Input: part model. Units: mm. Frame: model coordinates. A direction names the side the tool comes from. Coordinates: 2 decimals unless noted, no trailing zeros. Loops run counter-clockwise (first coordinate to the right, second up) from the corner with the lowest first, then second, coordinate; pieces in that order, holes last. Notation, with made-up numbers: (-4, -7) - (34, -7) arc R21 ccw to (34, 26) - close; hole circle Ø5 at (-14, 87.5). An arc over 180 degrees is marked (long way). Use one line per item in the form item = value.
from build123d import *

# Parameters (mm, degrees)
SKETCH1_W           = 0.508
SKETCH1_H           = 46.99
BOSS_EXTRUDE1_DEPTH = 6.35
SKETCH2_R           = 1
CUT_EXTRUDE1_DEPTH  = 6.35
SKETCH3_R           = 1
CUT_EXTRUDE2_DEPTH  = 6.35
SKETCH4_R           = 1
CUT_EXTRUDE3_DEPTH  = 2.54


with BuildPart() as part:
    # Sketch1 → Boss-Extrude1 (new body)
    with BuildSketch(Plane.XY):
        with Locations((0.254, 23.495)):
            Rectangle(SKETCH1_W, SKETCH1_H)
        Polygon((0, 46.99), (0.508, 46.99), (5.588, 67.31), (5.08, 67.31), align=None)
        Polygon((5.588, -20.32), (0.508, 0), (0, 0), (5.08, -20.32), align=None)
    extrude(amount=BOSS_EXTRUDE1_DEPTH)

    # Sketch2 → Cut-Extrude1 (cut)
    with BuildSketch(Plane.ZY):
        with Locations((3.175, 3.048)):
            Circle(SKETCH2_R)
        with Locations((3.175, 15.748)):
            Circle(SKETCH2_R)
        with Locations((3.175, 43.942)):
            Circle(SKETCH2_R)
        with Locations((3.175, 31.242)):
            Circle(SKETCH2_R)
    extrude(amount=-CUT_EXTRUDE1_DEPTH, mode=Mode.SUBTRACT)

    # Sketch3 → Cut-Extrude2 (cut)
    with BuildSketch(Plane(origin=(-11.056470588, 2.764117647, 0), x_dir=(0, 0, 1), z_dir=(-0.9701425001453319, 0.24253562503633325, 0))):
        with Locations(Location((3.175, 63.53237266, 0), (0, 0, 270))):
            Circle(SKETCH3_R)
    extrude(amount=-CUT_EXTRUDE2_DEPTH, mode=Mode.SUBTRACT)

    # Sketch4 → Cut-Extrude3 (cut)
    with BuildSketch(Plane(origin=(0.478117647, 0.119529412, 0), x_dir=(0, 0, -1), z_dir=(0.9701425001453319, 0.24253562503633308, 0))):
        with Locations(Location((-3.175, -17.945376578, 0), (0, 0, 90))):
            Circle(SKETCH4_R)
    extrude(amount=-CUT_EXTRUDE3_DEPTH, mode=Mode.SUBTRACT)


solid = part.part
Q1. Ray query, line 1 along X through (y, z) = (26.5, 1); line 2 along X through (y, z) = (-6.5, 3) (3 decimals). Return the intervals inside material, ascending. Write a range as [from, to].
Check values:
line_1 = [0, 0.51]
line_2 = [1.625, 2.133]
Q2. Cut plane C-C, the plane y = -3. Return loops of the section in (x, z), then the cut area to 3 significant figures.
Check values:
outline = (0.75, 0) - (1.26, 0) - (1.26, 6.35) - (0.75, 6.35) - close
area = 3.23 mm²
Q3. Cut plane A-A, the plane z = 1. Return loops of the section in (x, y), then the cut area to 3 significant figures.
Check values:
outline = (0, 0) - (5.08, -20.32) - (5.59, -20.32) - (0.51, 0) - (0.51, 46.99) - (5.59, 67.31) - (5.08, 67.31) - (0, 46.99) - close
area = 44.5 mm²
Q4. Pull-direction query (Z, two-part tool) for faces 3 (the cylindrical face through (0.25, 2.07, 2.96)), 4 (the flat face through (0.3, 23.7, 0)), 5 (the flat face through (2.5, -10, 3.1)), 6 (the flat face through (0.3, 23.7, 6.35)); classes: pulls with the +Z half, pulls with the -Z half, needs draft (parallel to the pull), parting line crosses it, or undercut.
Check values:
face_3 = undercut
face_4 = pulls with the -Z half
face_5 = needs draft
face_6 = pulls with the +Z half
Q5. Cut plane B-B, the plane x = 2.7. Return loops of the section in (y, z).
Check values:
outline = (-10.8, 0) - (-8.77, 0) - (-8.77, 6.35) - (-10.8, 6.35) - close; (55.76, 0) - (57.79, 0) - (57.79, 6.35) - (55.76, 6.35) - close
Q6. Set-up query: faces 1 (the flat face through (0.508, 23, 3)), 2 (the cylindrical face through (0.25, 44.933, 3.045)). Return all of +Z, -Z, +X, -X, +Y, -Y with unobstructed straight access to the full face (end or side cutting, diameter ignored); none if empty.
Check values:
face_1 = +Z, -Z, +X
face_2 = +X, -X
Q7. First-contact query: P1, Ø3, axis at y = 31.242, z = 3.175, coming from the -X side; P2, Ø1.5, axis at y = 56, z = 3.5, coming from the +X side; P3, Ø2, axis at y = -9.5, z = 3.5, coming from the +X side; P4, Ø1, axis at y = -8, z = 1.5, coming from the -X side (3 decimals). Flat tips, straight axial feed; report the tip coordinate or a pass-through.
Check values:
P1 = 0
P2 = 2.95
P3 = 3.13
P4 = 1.875
